Geometry: final body of the model. Coordinates: model frame, mm. Face numbers are marked on the shaded views. A direction names the side the tool comes from. Give positions to 0.01 mm unless a question says otherwise; leave off trailing zeros. Order: outer loops, then holes, each group sorted by start corner. A loop starts at its lowest first (then second) coordinate and runs counter-clockwise, first axis right, second up. Notation, with made-up numbers: M 48,69 L 104,69 A27 cw 104,93 Z; hole C -35,46 d4. An arc over 180 degrees is marked long. One line per item, written item: value. Start each with the question number.
```python
from build123d import *

# Parameters (mm, degrees)
ESBO_O1_R                    = 35
RESSALTO_EXTRUS_O1_DEPTH     = 50
FURO_ROSCADO_DE_M101_D       = 8.5
FURO_ROSCADO_DE_M101_DEPTH   = 27.5
FURO_ROSCADO_DE_M101_TIP     = 2.553657631
FUROS_GUIA_COM_10_0MM1_D     = 10
FUROS_GUIA_COM_10_0MM1_DEPTH = 27.5
FUROS_GUIA_COM_10_0MM1_TIP   = 3.004303095


with BuildPart() as part:
    # Esboço1 → Ressalto-extrusão1 (new body)
    with BuildSketch(Plane.XY):
        with Locations(Location((0, -240, 0), (0, 0, 180))):
            Circle(ESBO_O1_R)
    extrude(amount=RESSALTO_EXTRUS_O1_DEPTH)

    # Furo roscado de M101
    with Locations(Plane(origin=(0, 0, 0), x_dir=(-1, 0, 0), z_dir=(0, 0, -1))):
        with Locations((0, -220), (17.320508076, -250), (-17.320508076, -250)):
            Hole(FURO_ROSCADO_DE_M101_D / 2, depth=FURO_ROSCADO_DE_M101_DEPTH)
            with Locations((0, 0, -(FURO_ROSCADO_DE_M101_DEPTH + FURO_ROSCADO_DE_M101_TIP / 2))):  # 118° drill point
                Cone(0, FURO_ROSCADO_DE_M101_D / 2, FURO_ROSCADO_DE_M101_TIP, mode=Mode.SUBTRACT)

    # Furos-guia com Ø10.0mm1
    with Locations(Plane(origin=(0, 0, 0), x_dir=(-1, 0, 0), z_dir=(0, 0, -1))):
        with Locations((20, -230), (-20, -230)):
            Hole(FUROS_GUIA_COM_10_0MM1_D / 2, depth=FUROS_GUIA_COM_10_0MM1_DEPTH)
            with Locations((0, 0, -(FUROS_GUIA_COM_10_0MM1_DEPTH + FUROS_GUIA_COM_10_0MM1_TIP / 2))):  # 118° drill point
                Cone(0, FUROS_GUIA_COM_10_0MM1_D / 2, FUROS_GUIA_COM_10_0MM1_TIP, mode=Mode.SUBTRACT)


solid = part.part
```
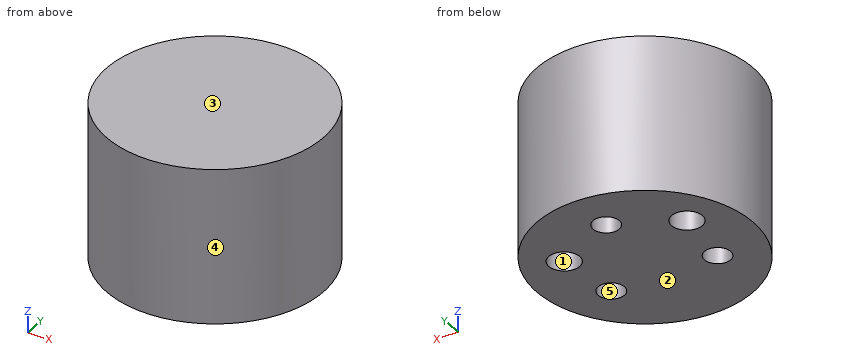
Q1. Section query A-A on z = 18.5. Return loops of the section in (x, y).
Q2. Contact query for flat-ended pins moving along their axis: pin 1 (10 mm diameter, centred on y = -225.5, z = 24.5, fed in from -X); pin 2 (1.5 mm diameter, centred on x = 17.5, y = -221.5, fed in from -Z); pin 3 (5 mm diameter, centred on x = -7.5, z = 12, fed in from -Y); pin 4 (8 mm diameter, centred on x = 6, z = 21.5, fed in from -Y). Output: stop coordinate, or through.
Q3. Mould query, pull axis Y, two halves, no side actions, for the marked faces 3, 4 and 5. Classes: +Y half, -Y half, draft (parallel to the pull), parting line (faces both ways), or undercut.
Q4. Set-up query: the marked faces 1 and 2. Return all of +Z, -Z, +X, -X, +Y, -Y with unobstructed straight access to the full face (end or side cutting, diameter ignored); none if empty.
Q5. Ray query, line 1 along X through (y, z) = (-250, 18.25); line 2 along Y through (x, z) = (17, 27.5); line 3 along Y through (x, z) = (-20.5, 25). Return the intervals inside material, ascending. Write a range as [from, to].
Q6. Section query B-B on z = 39. Return loops of the section in (x, y), and give its area (3 significant figures).
Q7. Section query D-D on y = -266. Return loops of the section in (x, z), and give its area (3 significant figures).
Q8. Section query C-C on x = -11. Return loops of the section in (y, z).
Results below:
1. outline: C 0,-240 d70; hole C -20,-230 d10; hole C -17.32,-250 d8.5; hole C 0,-220 d8.5; hole C 17.32,-250 d8.5; hole C 20,-230 d10
2. pin 1: x = -33.69
2. pin 2: z = 0
2. pin 3: y = -274.64
2. pin 4: y = -274.94
3. face 3: draft
3. face 4: parting line
3. face 5: undercut
4. face 1: -Z
4. face 2: -Z, +X, -X, +Y, -Y
5. line 1: [-33.54, -21.57], [-13.07, 13.07], [21.57, 33.54]
5. line 2: [-270.59, -254.24], [-245.76, -234], [-226, -209.41]
5. line 3: [-268.37, -252.82], [-247.18, -234.97], [-225.03, -211.63]
6. outline: C 0,-240 d70
6. area: 3,850 mm2
7. outline: M -23.43,0 L 23.43,0 L 23.43,50 L -23.43,50 Z
7. area: 2,340 mm2
8. outline: M -273.23,0 L -206.77,0 L -206.77,50 L -273.23,50 Z
